The model under review builds one solid part; all positions refer to its coordinate system, in mm. Face numbers are marked on the shaded views. Round coordinates to 2 decimals unless told otherwise and drop trailing zeros. Loops run counter-clockwise (first coordinate to the right, second up) from the corner with the lowest first, then second, coordinate; pieces in that order, holes last. Notation, with made-up numbers: M 64,1.25 L 118,1.25 A33 cw 118,30.25 Z; hole C -24,-18 d4. An arc over 180 degrees is marked long. Return JSON: item names as keys, results as strings. Group by question number.
Q1. Draft analysis for pull direction Y (two halves, no side actions). For the marked faces 1, 2 and 3, state which applies: pulls with the +Y half, pulls with the -Y half, needs draft (parallel to the pull), parting line crosses it, or undercut.
Q2. Consider section D-D (z = 126). State the section outline as (x, y) points, and give its area (3 significant figures).
Q3. To check wall thickness, follow line 1 along X through (y, z) = (196, 0); line 2 along X through (y, z) = (474.5, 0); line 3 along Y through (x, z) = (52.5, -107.5). State the ranges of each line that lie inside material, in increasing order.
Q4. Consider section B-B (z = 0). State the section outline as (x, y) points.
Q5. Consider section C-C (y = 371). State the section outline as (x, z) points.
Q6. Consider section A-A (x = 0). State the section outline as (y, z) points, and give its area (3 significant figures).
Q7. Clearance check with flat-ended pins moving along their axes: pin 1 Ø5 at (y, z) = (304, 72) entering from +X; pin 2 Ø5 at (x, y) = (116, 273) entering from -Z; pin 3 Ø8 at (x, z) = (-82, -122) entering from -Y; pin 4 Ø1 at (y, z) = (336, -25) entering from +X. State where each tip first meets the part, or that it passes through.
from build123d import *

# Parameters (mm, degrees)
RECEPTACLE_FLOOR_SKETCH_R   = 185
RECEPTACLE_FLOOR_SKETCH_R_2 = 12.5
RECEPTACLE_FLOOR_DEPTH      = 6
RECEPTACLE_WALL_SKETCH_R    = 180
RECEPTACLE_WALL_SKETCH_R_2  = 176
RECEPTACLE_WALL_DEPTH       = 480
POT_START                   = 470
POT_SEAT_LEDGE_SKETCH_R     = 177
POT_SEAT_LEDGE_SKETCH_R_2   = 170
POT_SEAT_LEDGE_DEPTH        = 10


with BuildPart() as part:
    # Receptacle Floor Sketch → Receptacle Floor (new body)
    with BuildSketch(Plane(origin=(0, 0, 0), x_dir=(1, 0, 0), z_dir=(0, 1, 0))):
        with Locations(Location((0, 0, 0), (0, 0, 270))):
            Circle(RECEPTACLE_FLOOR_SKETCH_R)
        with Locations(Location((0, 0, 0), (0, 0, 270))):
            Circle(RECEPTACLE_FLOOR_SKETCH_R_2, mode=Mode.SUBTRACT)
    extrude(amount=RECEPTACLE_FLOOR_DEPTH)

    # Receptacle Wall Sketch → Receptacle Wall (add)
    with BuildSketch(Plane(origin=(0, 0, 0), x_dir=(1, 0, 0), z_dir=(0, 1, 0))):
        with Locations(Location((0, 0, 0), (0, 0, 270))):
            Circle(RECEPTACLE_WALL_SKETCH_R)
        with Locations(Location((0, 0, 0), (0, 0, 270))):
            Circle(RECEPTACLE_WALL_SKETCH_R_2, mode=Mode.SUBTRACT)
    extrude(amount=RECEPTACLE_WALL_DEPTH)

    # Pot Seat Ledge Sketch → Pot Seat Ledge (add)
    with BuildSketch(Plane(origin=(0, 0, 0), x_dir=(1, 0, 0), z_dir=(0, 1, 0)).offset(POT_START)):
        Circle(POT_SEAT_LEDGE_SKETCH_R)
        with Locations(Location((0, 0, 0), (0, 0, 270))):
            Circle(POT_SEAT_LEDGE_SKETCH_R_2, mode=Mode.SUBTRACT)
    extrude(amount=POT_SEAT_LEDGE_DEPTH)


solid = part.part
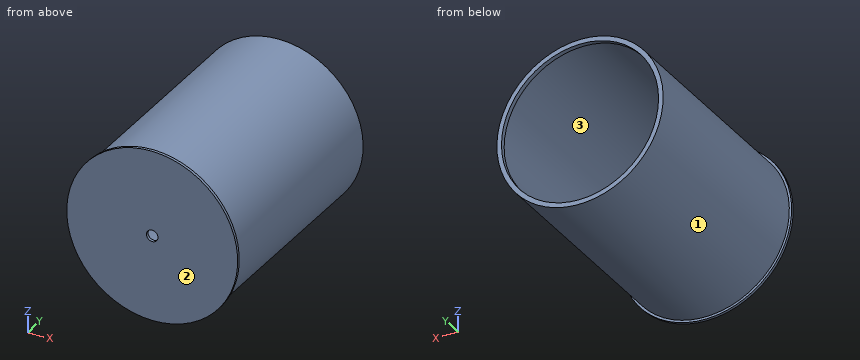
Values:
{
 "1": {"face 1": "needs draft", "face 2": "pulls with the -Y half", "face 3": "undercut"},
 "2": {"outline": "M -135.46,0 L 135.46,0 L 135.46,6 L 128.55,6 L 128.55,480 L 114.12,480 L 114.12,470 L 122.88,470 L 122.88,6 L -122.88,6 L -122.88,470 L -114.12,470 L -114.12,480 L -128.55,480 L -128.55,6 L -135.46,6 Z", "area": "7,170 mm2"},
 "3": {"line 1": "x = -180 to -176, 176 to 180", "line 2": "x = -180 to -170, 170 to 180", "line 3": "y = 0 to 6"},
 "4": {"outline": "M -185,0 L -12.5,0 L -12.5,6 L -176,6 L -176,470 L -170,470 L -170,480 L -180,480 L -180,6 L -185,6 Z; M 12.5,0 L 185,0 L 185,6 L 180,6 L 180,480 L 170,480 L 170,470 L 176,470 L 176,6 L 12.5,6 Z"},
 "5": {"outline": "C 0,0 d360; hole C 0,0 d352"},
 "6": {"outline": "M 0,-185 L 6,-185 L 6,-180 L 480,-180 L 480,-170 L 470,-170 L 470,-176 L 6,-176 L 6,-12.5 L 0,-12.5 Z; M 0,12.5 L 6,12.5 L 6,176 L 470,176 L 470,170 L 480,170 L 480,180 L 6,180 L 6,185 L 0,185 Z", "area": "5,980 mm2"},
 "7": {"pin 1": "stops at x = 166.04", "pin 2": "stops at z = -139.71", "pin 3": "stops at y = 0", "pin 4": "stops at x = 178.32"}
}
